Check sheet for the drawn part. Datum: minimum x, y, z corner. Units: mm. A direction names the side the tool comes from. Coordinates: 2 decimals unless noted, no trailing zeros. Order: outer loops, then holes, each group sorted by start corner. A loop starts at its lowest first (then second) coordinate and runs counter-clockwise, first axis right, second up. Notation, with made-up numbers: M 79,88.5 L 113,88.5 A23 ccw 113,99.5 Z; hole C 10,-15.75 d5. An arc over 180 degrees is marked long. Return JSON: item names as keys, results as strings. Group by question number.
Q1. Access from +Z, -Z, +X, -X, +Y, -Y to the whole of each face (thin tool, end or side, straight path). Record for the marked faces 1, 2 and 3.
Q2. Thickness scan on probe 1 along Z at (x, y) = (53, 43.5); probe 2 along Z at (x, y) = (44, 84); probe 3 along Y at (x, z) = (44, 10). Record the ranges inside material, lowest first.
Q3. Section check D-D, the plane z = 62. Enter the section's corners in (x, y), then the cut area to 3 significant figures.
Q4. Section check C-C, the plane y = 72. Enter the section's corners in (x, z).
Q5. Mould release check, pull along Z, two halves, no side actions. Record for the marked faces 4, 5 and 6: pulls with the +Z half, pulls with the -Z half, needs draft (parallel to the pull), parting line crosses it, or undercut.
Q6. Section check B-B, the plane x = 44. Enter the section's corners in (y, z), then the cut area to 3 significant figures.
Q7. Section check A-A, the plane y = 44. Enter the section's corners in (x, z), then the cut area to 3 significant figures.
Q8. Go/stop test with flat-tipped pins: pin 1 Ø2 at (x, z) = (9.5, 82.5) entering from -Y; pin 2 Ø2 at (x, y) = (20, 10) entering from -Z; pin 3 Ø1.5 at (x, z) = (29.5, 87.5) entering from -Y; pin 4 Ø6 at (x, z) = (24, 92.5) entering from +Y. Record where each tip stops, or that it passes through.
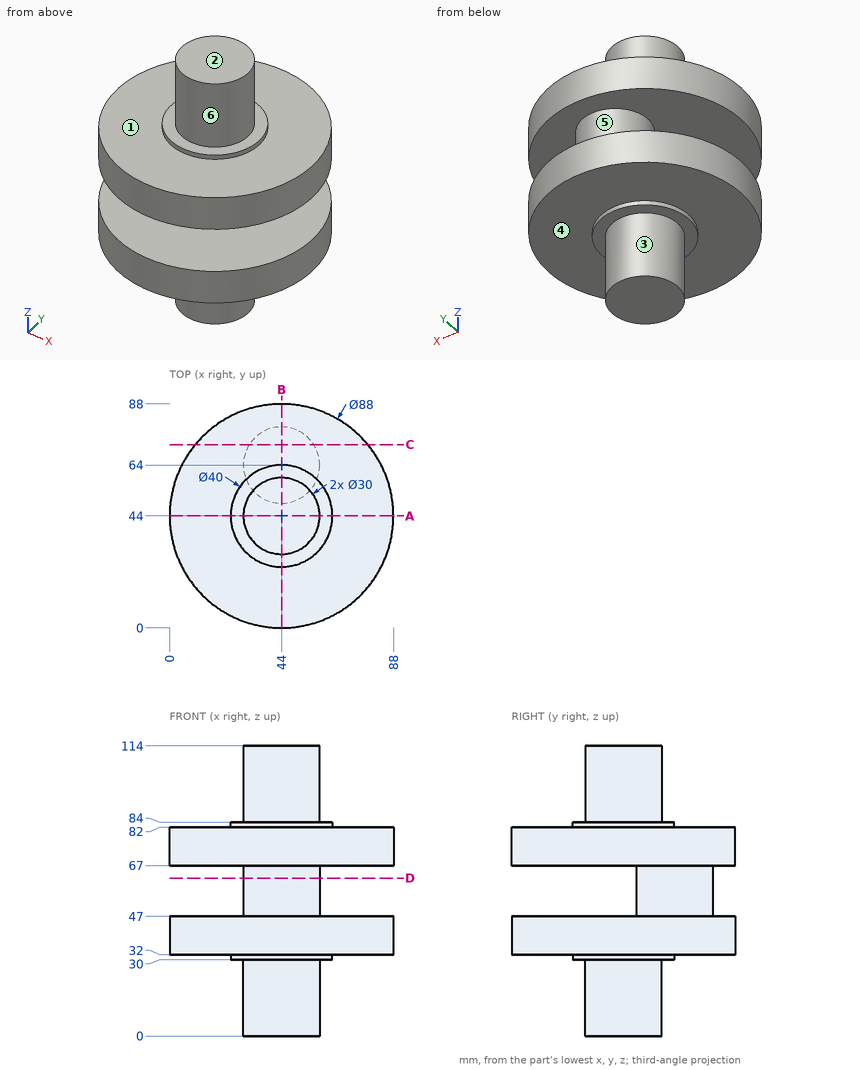
Numbers:
{
 "1": {"face 1": "+Z", "face 2": "+Z, +X, -X, +Y, -Y", "face 3": "-Z"},
 "2": {"probe 1": "z = 0 to 47, 67 to 114", "probe 2": "z = 32 to 47, 67 to 82", "probe 3": "y = 29 to 59"},
 "3": {"outline": "C 44,64 d30", "area": "707 mm2"},
 "4": {"outline": "M 10.06,32 L 77.94,32 L 77.94,47 L 56.69,47 L 56.69,67 L 77.94,67 L 77.94,82 L 10.06,82 L 10.06,67 L 31.31,67 L 31.31,47 L 10.06,47 Z"},
 "5": {"face 4": "pulls with the -Z half", "face 5": "undercut", "face 6": "needs draft"},
 "6": {"outline": "M 0,32 L 24,32 L 24,30 L 29,30 L 29,0 L 59,0 L 59,30 L 64,30 L 64,32 L 88,32 L 88,47 L 79,47 L 79,67 L 88,67 L 88,82 L 64,82 L 64,84 L 59,84 L 59,114 L 29,114 L 29,84 L 24,84 L 24,82 L 0,82 L 0,67 L 49,67 L 49,47 L 0,47 Z", "area": "5,200 mm2"},
 "7": {"outline": "M 0,32 L 24,32 L 24,30 L 29,30 L 29,0 L 59,0 L 59,30 L 64,30 L 64,32 L 88,32 L 88,47 L 0,47 Z; M 0,67 L 88,67 L 88,82 L 64,82 L 64,84 L 59,84 L 59,114 L 29,114 L 29,84 L 24,84 L 24,82 L 0,82 Z", "area": "4,600 mm2"},
 "8": {"pin 1": "stops at y = 15.63", "pin 2": "stops at z = 32", "pin 3": "stops at y = 38.01", "pin 4": "passes through"}
}
